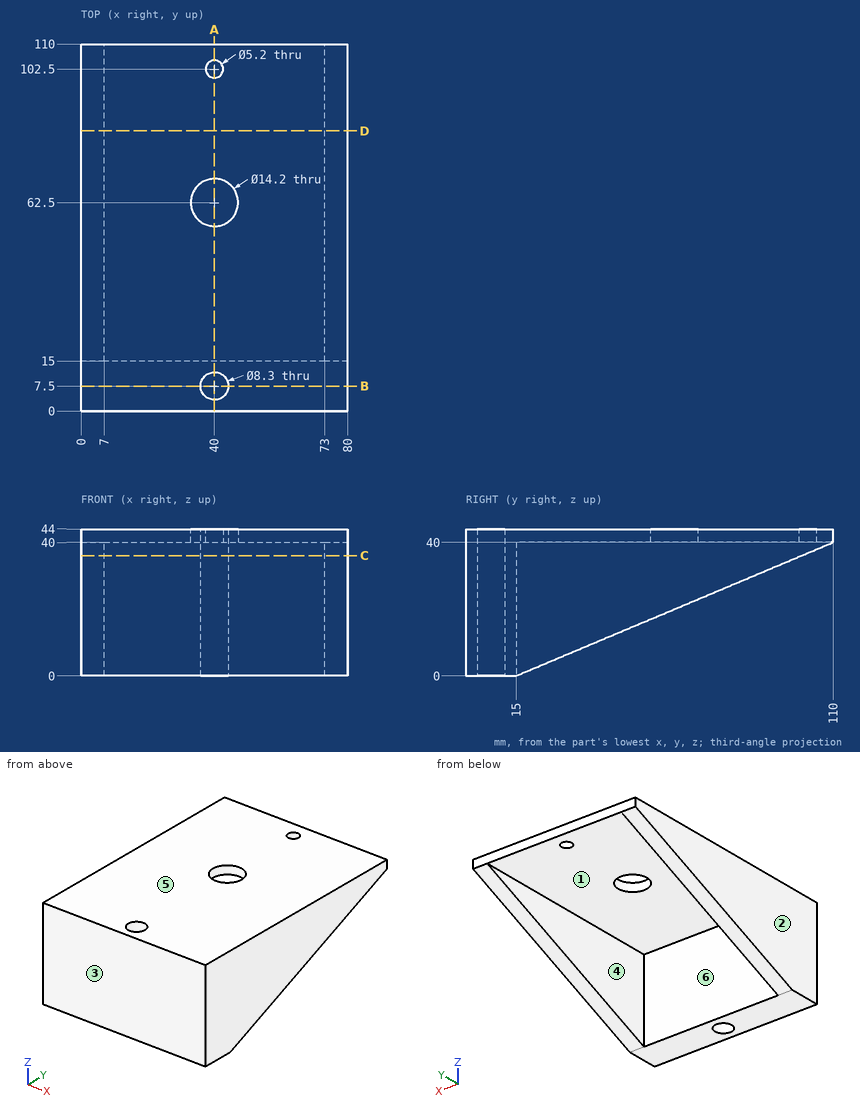
Job drawing, mm, ordinate dimensions from the low corner. One solid piece. A direction names the side the tool comes from. Round coordinates to 2 decimals unless told otherwise and drop trailing zeros. Write each loop counter-clockwise with the first axis right and the second up, starting at its lowest first coordinate (ties: lowest second). Pieces come first, ordered by that corner, then holes.
1) Band-saw the part on D-D, the plane y = 84. List the corners of the cut face in (x, z), and give its area (3 significant figures).
2) Pin check, flat tips, straight feed: pin 1 (5 mm diameter, centred on x = 40, y = 7.5, fed in from -Z) (3 decimals); pin 2 (20 mm diameter, centred on x = 23.5, z = 23, fed in from +Y); pin 3 (1 mm diameter, centred on x = 45.5, y = 25.5, fed in from -Z). Stop position of each tip, or through.
3) Band-saw the part on A-A, the plane x = 40. List the corners of the cut face in (y, z).
4) Mould opens along X. For the marked faces 1, 2, 3 and 4 say: +X half, -X half, draft (parallel to the pull), parting line (faces both ways), or undercut.
5) Drill centre lines: probe 1 along Y at (x, z) = (40, 41.95); probe 2 along X at (y, z) = (19.5, 38); probe 3 along Y at (x, z) = (40, 34). Where is each one in solid material? Low to high.
6) 3-axis set-ups, long thin cutter, end or side, ignore diameter. For the marked faces 5 and 6: which of +Z, -Z, +X, -X, +Y, -Y reach the whole face in a straight line?
7) Band-saw the part on B-B, the plane y = 7.5. List the corners of the cut face in (x, z), and give its area (3 significant figures).
8) Band-saw the part on C-C, the plane z = 36. List the corners of the cut face in (x, y), and give its area (3 significant figures).
Ans:
1. outline: (0, 29.05) - (7, 29.05) - (7, 40) - (73, 40) - (73, 29.05) - (80, 29.05) - (80, 44) - (0, 44) - close
1. area: 473 mm2
2. pin 1: passes through
2. pin 2: stops at y = 15
2. pin 3: stops at z = 40
3. outline: (0, 0) - (3.35, 0) - (3.35, 44) - (0, 44) - close; (11.65, 0) - (15, 0) - (15, 40) - (55.4, 40) - (55.4, 44) - (11.65, 44) - close; (69.6, 40) - (99.9, 40) - (99.9, 44) - (69.6, 44) - close; (105.1, 40) - (110, 40) - (110, 44) - (105.1, 44) - close
4. face 1: undercut
4. face 2: -X half
4. face 3: draft
4. face 4: undercut
5. probe 1: y = 0 to 3.35, 11.65 to 55.4, 69.6 to 99.9, 105.1 to 110
5. probe 2: x = 0 to 7, 73 to 80
5. probe 3: y = 0 to 3.35, 11.65 to 15
6. face 5: +Z, +X, -X, +Y, -Y
6. face 6: -Z, +Y
7. outline: (0, 0) - (35.85, 0) - (35.85, 44) - (0, 44) - close; (44.15, 0) - (80, 0) - (80, 44) - (44.15, 44) - close
7. area: 3,150 mm2
8. outline: (0, 0) - (80, 0) - (80, 100.5) - (73, 100.5) - (73, 15) - (7, 15) - (7, 100.5) - (0, 100.5) - close; hole circle Ø8.3 at (40, 7.5)
8. area: 2,340 mm2
